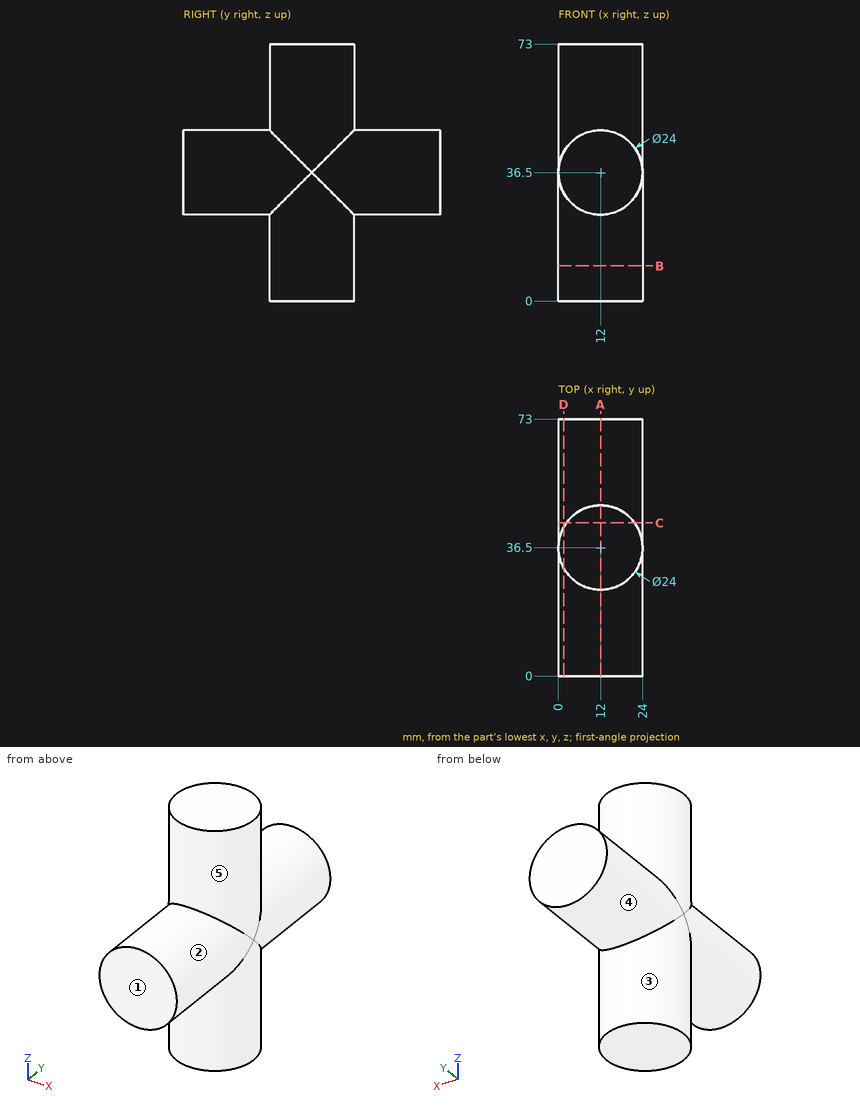
Here's the drawing with two shaded views (mm, measured from the low corner). I have some questions. A direction names the side the tool comes from. Round coordinates to 2 decimals unless told otherwise and drop trailing zeros. Loops run counter-clockwise (first coordinate to the right, second up) from the corner with the lowest first, then second, coordinate; pieces in that order, holes last. Notation, with made-up numbers: (30.25, -25) -> (81.25, -25) arc R34 ccw to (81.25, 5) -> close; hole circle Ø9 at (13.5, -5). An arc over 180 degrees is marked (long way). Answer as CSV lines item,"result". Start each with the question number.
1. I'm going to push flat-ended pins straight in: P1, Ø5, axis at y = 52.5, z = 26.5, coming from the -X side; P2, Ø4, axis at x = 9, z = 58, coming from the -Y side; P3, Ø1.5, axis at x = 2.5, z = 23.5, coming from the -Y side; P4, Ø2, axis at x = 12, y = 35.5, coming from the -Z side. Where does each tip first touch, or does it pass through?
2. I need wall thicknesses on probe 1 along Z at (x, y) = (11.5, 20); probe 2 along Y at (x, z) = (11.75, 5); probe 3 along X at (y, z) = (32.5, 67). Which ranges of each line are inside material? Lowest first, please. Write a range as from..to.
3. If we mould it in two halves opening along X, with no side actions, what happens to the marked faces 1 and 2? For each: pulls with the +X half, pulls with the -X half, needs draft (parallel to the pull), parting line crosses it, or undercut.
4. Imagine slicing it at B-B on z = 10. Write out the boundary of the cut face in (x, y), plus the area to 3 significant figures.
5. Imagine slicing it at D-D on x = 1.5. Write out the boundary of the cut face in (y, z).
6. Imagine slicing it at A-A on x = 12. Write out the boundary of the cut face in (y, z), plus the area to 3 significant figures.
7. For the marked faces 3, 4 and 5, which set-ups out of +Z, -Z, +X, -X, +Y, -Y let a thin tool reach every point of the face, with its end or its side?
8. Imagine slicing it at C-C on y = 43.5. Write out the boundary of the cut face in (x, z).
Solution:
1,P1,"x = 2.63"
1,P2,"y = 24.54"
1,P3,"y = 28.29"
1,P4,"z = 0"
2,probe 1,"24.51..48.49"
2,probe 2,"24.5..48.5"
2,probe 3,"0.69..23.31"
3,face 1,"needs draft"
3,face 2,"parting line crosses it"
4,outline,"circle Ø24 at (12, 36.5)"
4,area,"452 mm²"
5,outline,"(0, 30.69) -> (30.69, 30.69) -> (30.69, 0) -> (42.31, 0) -> (42.31, 30.69) -> (73, 30.69) -> (73, 42.31) -> (42.31, 42.31) -> (42.31, 73) -> (30.69, 73) -> (30.69, 42.31) -> (0, 42.31) -> close"
6,outline,"(0, 24.5) -> (24.5, 24.5) -> (24.5, 0) -> (48.5, 0) -> (48.5, 24.5) -> (73, 24.5) -> (73, 48.5) -> (48.5, 48.5) -> (48.5, 73) -> (24.5, 73) -> (24.5, 48.5) -> (0, 48.5) -> close"
6,area,"2,930 mm²"
7,face 3,"-Z"
7,face 4,"+Y"
7,face 5,"+Z"
8,outline,"(2.25, 0) -> (21.75, 0) -> (21.75, 29.5) arc R12 ccw to (21.75, 43.5) -> (21.75, 73) -> (2.25, 73) -> (2.25, 43.5) arc R12 ccw to (2.25, 29.5) -> close"
